Source: CAD feature listing. Evaluate the final solid. Frame: model axes, mm. A direction names the side the tool comes from. Coordinates: 2 decimals unless noted, no trailing zeros. Write each loop counter-clockwise with the first axis right and the second up, starting at its lowest first coordinate (ties: lowest second). Pieces come first, ordered by that corner, then holes. Notation, with made-up numbers: (68.5, -0.75) -> (109.5, -0.75) arc R12 cw to (109.5, 13.25) -> close; hole circle Ø1 at (-15, 69). An arc over 180 degrees is marked (long way). Write item = value, one per line.
from build123d import *

# Parameters (mm, degrees)
BOSS_EXTRUDE1_DEPTH = 8
BOSS_EXTRUDE2_START = 1.5
BOSS_EXTRUDE2_DEPTH = 1.5
SKETCH4_R           = 2.425
SKETCH4_R_2         = 1.625
EXTRUDE_THIN1_DEPTH = 3
FILLET1_R           = 1.5


with BuildPart() as part:
    # Sketch1 → Boss-Extrude1 (new body)
    with BuildSketch(Plane(origin=(0, 0, 0), x_dir=(1, 0, 0), z_dir=(0, 1, 0))):
        Polygon((-7.130275824, 0), (-3.565137912, -6.175), (3.565137912, -6.175), (7.130275824, 0), (3.565137912, 6.175), (-3.565137912, 6.175), align=None)
        with BuildLine():
            Line((-1.15, 1.14809625), (-1.15, -1.14809625))
            ThreePointArc((-1.15, -1.14809625), (1.625, 0), (-1.15, 1.14809625))
        make_face(mode=Mode.SUBTRACT)
    extrude(amount=BOSS_EXTRUDE1_DEPTH)

    # Sketch2 → Boss-Extrude2 (add)
    with BuildSketch(Plane.XZ.offset(BOSS_EXTRUDE2_START)):
        Polygon((-4.431163316, 7.675), (-8.862326632, 0), (-4.431163316, -7.675), (4.431163316, -7.675), (8.862326632, 0), (4.431163316, 7.675), align=None)
        with BuildLine():
            Line((-1.15, -1.14809625), (-1.15, 1.14809625))
            ThreePointArc((-1.15, 1.14809625), (1.625, 0), (-1.15, -1.14809625))
        make_face(mode=Mode.SUBTRACT)
    extrude(amount=-BOSS_EXTRUDE2_DEPTH)

    # Sketch4 → Extrude-Thin1 (add)
    with BuildSketch(Plane(origin=(0, 8, 0), x_dir=(1, 0, 0), z_dir=(0, 1, 0))):
        Circle(SKETCH4_R)
        Circle(SKETCH4_R_2, mode=Mode.SUBTRACT)
    extrude(amount=EXTRUDE_THIN1_DEPTH)

    # Fillet1
    fillet1_edges = [part.edges().sort_by_distance(p)[0] for p in [
        (0, 8, 6.175),
        (-3.565137912, 4, -6.175),
        (3.565137912, 4, -6.175),
        (7.130275824, 4, 0),
        (3.565137912, 4, 6.175),
        (-3.565137912, 4, 6.175),
        (-7.130275824, 4, 0),
        (5.347706868, 8, 3.0875),
        (5.347706868, 8, -3.0875),
        (0, 8, -6.175),
        (-5.347706868, 8, -3.0875),
        (-2.425, 8, 0),
        (-5.347706868, 8, 3.0875),
    ]]
    fillet(fillet1_edges, radius=FILLET1_R)


solid = part.part
1) First-contact query: pin 1 Ø6 at (x, y) = (-0.5, 4) entering from -Z (3 decimals); pin 2 Ø2 at (y, z) = (0, -5.5) entering from -X; pin 3 Ø6 at (x, y) = (-5.5, 4) entering from +Z (3 decimals). Flat tips, straight axial feed; report the tip coordinate or a pass-through.
Answer block:
pin_1 = -6.175
pin_2 = -6.26
pin_3 = 6.175
2) Reachability of faces 1 (the flat face through (3, 8, -3)), 2 (the cylindrical face through (-3.46, 3.3, -5.97)), 3 (the cylindrical face through (3.4, 3.3, 6)) from +Z, -Z, +X, -X, +Y, -Y: full face, straight path, thin tool, end or side. Return the list, or none.
Answer block:
face_1 = +Y
face_2 = -Z, -X, +Y
face_3 = +Z, +X, +Y
3) Cut plane A-A, the plane y = 4.75. Output: boundary loops of the cut face in (x, z) (3 decimals).
Answer block:
outline = (-6.697, -0.75) -> (-3.998, -5.425) arc R1.5 ccw to (-2.699, -6.175) -> (2.699, -6.175) arc R1.5 ccw to (3.998, -5.425) -> (6.697, -0.75) arc R1.5 ccw to (6.697, 0.75) -> (3.998, 5.425) arc R1.5 ccw to (2.699, 6.175) -> (-2.699, 6.175) arc R1.5 ccw to (-3.998, 5.425) -> (-6.697, 0.75) arc R1.5 ccw to start; hole (-1.15, -1.148) arc R1.625 ccw (long way) to (-1.15, 1.148) -> close
4) Material intervals for probe 1 along Z at (x, y) = (0, 4.75) (3 decimals); probe 2 along X at (y, z) = (6, 0) (3 decimals); probe 3 along Y at (x, z) = (-6, 3), sorted ascending. Write a range as [from, to].
Answer block:
probe_1 = [-6.175, -1.625], [1.625, 6.175]
probe_2 = [-6.898, -1.15], [1.625, 6.898]
probe_3 = [-1.5, 0]
5) Pull-direction query (X, two-part tool) for faces 4 (the cylindrical face through (-3.46, 3.3, 5.97)), 5 (the flat face through (-1.15, 3, 0)), 6 (the flat face through (5.37, 3.2, -3.05)); classes: +X half, -X half, draft (parallel to the pull), parting line (faces both ways), or undercut.
Answer block:
face_4 = -X half
face_5 = undercut
face_6 = +X half
